Autodesk Inventor part; units mm, degrees
sketch "Sketch1" plane through (0, 0, 0) normal (0, 0, 1) x (1, 0, 0)
  circle A0 centre (0, 0) radius 12.7
  circle A1 centre (0, 0) radius 50.8
  dimension "d0" = 101.6
  dimension "d1" = 25.4
extrude "Extrusion1" add sketch "Sketch1" along normal mid plane 50.8
sketch "Sketch2" plane through (0, 0, -25.4) normal (0, 0, -1) x (-1, 0, 0)
  circle A0 centre (0, 0) radius 40 construction
  circle A1 centre (0, 0) radius 12.7 construction
  line L0 (0, 0) -> (0, 40) construction
  dimension "d4" = 80
hole "Hole1" at (0, 40, -25.4) direction (0, 0, 1) diameter 8 end through all
pattern_circular "Circular Pattern1" count 6 over 360 about axis through (0, 0, -10) along (0, 0, 1) of "Hole1"
chamfer "Chamfer1" distance 2 angle 45 2 edges at (-50.8, 0, -25.4) (-50.8, 0, 25.4)
chamfer "Chamfer2" distance 1 angle 45 2 edges at (-12.7, 0, -25.4) (-12.7, 0, 25.4)
properties part number "Porsche_912_CV_Joint"
The listing builds one solid part. Answer for the finished solid, in the listing's coordinates (mm). Coordinates: 2 decimals unless noted, no trailing zeros. Write each loop counter-clockwise with the first axis right and the second up, starting at its lowest first coordinate (ties: lowest second). Pieces come first, ordered by that corner, then holes. Notation, with made-up numbers: (46, -37) - (55, -37) arc R30 cw to (55, -14) - close; hole circle Ø6 at (44, 33). An arc over 180 degrees is marked (long way). Return JSON: item names as keys, results as strings. Group by question number.
Q1. For a pull along X with two mould halves and no side action, classify faces 1 (the flat face through (10, -10, 25.4)), 2 (the conical face through (46.67, 14.7, -25.27)), 3 (the cylindrical face through (37.075, -23.174, 0.356)), 4 (the cylindrical face through (34.817, 23.996, 0.356)) as +X half, -X half, draft (parallel to the pull), parting line (faces both ways), or undercut.
Q2. Find the intervals of material crossed by line 1 along X through (y, z) = (18.5, 17); line 2 along Y through (x, z) = (-1.5, -4); line 3 along Y through (x, z) = (32.5, 11), in increasing order. Write a range as [from, to].
Q3. The part is cut by section B-B on z = 16. Write down the section's boundary in (x, y), and give its area (3 significant figures).
Q4. Flat-ended cylindrical pins translate along their axes: pin 1 Ø3 at (x, z) = (-19, 13) entering from -Y; pin 2 Ø8 at (x, z) = (13, 18.5) entering from +Y; pin 3 Ø5 at (y, z) = (35.5, -13) entering from -X. Find the tip coordinate at first contact, or state that the pin passes through.
Q5. The part is cut by section C-C on x = -35.5. State how many separate pieces and enclosed holes the cut face has, and give its area (3 significant figures).
Q6. The part is cut by section A-A on x = 0. Write down the section's boundary in (y, z), and give its area (3 significant figures).
Evaluation:
{
 "1": {"face 1": "draft", "face 2": "parting line", "face 3": "undercut", "face 4": "undercut"},
 "2": {"line 1": "x = [-47.31, -38.35], [-30.93, 30.93], [38.35, 47.31]", "line 2": "y = [-50.78, -43.71], [-36.29, -12.61], [12.61, 36.29], [43.71, 50.78]", "line 3": "y = [-39.04, -23.38], [-16.62, 16.62], [23.38, 39.04]"},
 "3": {"outline": "circle Ø101.6 at (0, 0); hole circle Ø8 at (-34.64, -20); hole circle Ø8 at (-34.64, 20); hole circle Ø25.4 at (0, 0); hole circle Ø8 at (0, -40); hole circle Ø8 at (0, 40); hole circle Ø8 at (34.64, -20); hole circle Ø8 at (34.64, 20)", "area": "7,300 mm2"},
 "4": {"pin 1": "stops at y = -47.69", "pin 2": "stops at y = 50", "pin 3": "stops at x = -38.62"},
 "5": {"separate pieces": "3", "enclosed holes": "0", "area": "2,890 mm2"},
 "6": {"outline": "(-50.8, -23.4) - (-48.8, -25.4) - (-44, -25.4) - (-44, 25.4) - (-48.8, 25.4) - (-50.8, 23.4) - close; (-36, -25.4) - (-13.7, -25.4) - (-12.7, -24.4) - (-12.7, 24.4) - (-13.7, 25.4) - (-36, 25.4) - close; (12.7, -24.4) - (13.7, -25.4) - (36, -25.4) - (36, 25.4) - (13.7, 25.4) - (12.7, 24.4) - close; (44, -25.4) - (48.8, -25.4) - (50.8, -23.4) - (50.8, 23.4) - (48.8, 25.4) - (44, 25.4) - close", "area": "3,050 mm2"}
}
